Design review of the part built by this model. Coordinates are the model's own, in mm. A direction names the side the tool comes from. Round coordinates to 2 decimals unless told otherwise and drop trailing zeros. Order: outer loops, then holes, each group sorted by start corner. A loop starts at its lowest first (then second) coordinate and runs counter-clockwise, first axis right, second up. Notation, with made-up numbers: M -29.5,-7 L 20.5,-7 A33 cw 20.5,25 Z; hole C -33,85 d4. An arc over 180 degrees is marked long. Use a Markdown table: item, result. Add a question column.
(1) Take a section at C-C (z = 0). Write out the cut boundary in (x, y) (3 decimals), then the cut area to 3 significant figures.
(2) Take a section at D-D (x = -12). Write out the cut boundary in (y, z) (1 decimal), then the cut area to 3 significant figures.
(3) To check wall thickness, follow probe 1 along X at (y, z) = (3.5, 11.5) (1 decimal); probe 2 along X at (y, z) = (7.5, -12) (1 decimal); probe 3 along X at (y, z) = (8.25, 10.5) (1 decimal). State the ranges of each line that lie inside material, in increasing order. Write a range as from..to.
(4) Machinability: for faces 4 (the face through (-7.937, 5, -19)), 5 (the face through (9.68, 4.7, 8.34)), 6 (the face through (-3.175, 5, -13)), which of the approach directions +Z, -Z, +X, -X, +Y, -Y give a long, thin tool a straight path to every point of the face, cutting with its end or side? Answer none if there is none.
(5) For pin 1 (4 mm diameter, centred on y = 3.5, z = -0.5, fed in from +X); pin 2 (3 mm diameter, centred on y = 4.76, z = -15.88, fed in from +X); pin 3 (3 mm diameter, centred on y = 5, z = -12.5, fed in from +X); pin 4 (1.3 mm diameter, centred on x = 13.5, y = 4.5, fed in from -Z) (3 decimals), all flat-tipped, find the tip position at first contact; note any pin that passes through.
(6) The part is to be moulded in two halves that separate along Z. For faces 1 (the face through (13.46, 2.407, 15.352)), 2 (the face through (11.112, 5.9, 18.2)), 3 (the face through (-6, 5, -22.225)), say which applies: released by +Z, released by -Z, zero draft, split by the parting line, or undercut.
(7) Take a section at B-B (x = 0). Write out the cut boundary in (y, z) (3 decimals).
```python
from build123d import *

# Parameters (mm, degrees)
BOSS_EXTRUDE1_DEPTH                   = 9.525
SKETCH2_W                             = 19.05
SKETCH2_H                             = 15.24
SKETCH2_W_2                           = 22.225
CUT_EXTRUDE1_DEPTH                    = 10.525
F_3_16_0_1875_CLEARANCE_DOWEL_HOLE1_D = 4.826
F_10_24_TAPPED_HOLE1_D                = 3.7973
F_10_24_TAPPED_HOLE1_DEPTH            = 9.525
FILLET1_R                             = 4.7625
FILLET2_R                             = 12.7


with BuildPart() as part:
    # Sketch1 → Boss-Extrude1 (new body)
    with BuildSketch(Plane(origin=(0, 0, 0), x_dir=(1, 0, 0), z_dir=(0, 1, 0))):
        Polygon((-3.175, 22.225), (-3.175, 6.985), (3.175, 6.985), (3.175, 22.225), (26.9875, 22.225), (26.9875, -22.225), (22.225, -22.225), (22.225, -6.985), (15.875, -6.985), (15.875, -22.225), (-15.875, -22.225), (-15.875, -6.985), (-22.225, -6.985), (-22.225, -22.225), (-26.9875, -22.225), (-26.9875, 22.225), align=None)
    extrude(amount=BOSS_EXTRUDE1_DEPTH)

    # Sketch2 → Cut-Extrude1 (cut, through all)
    with BuildSketch(Plane(origin=(0, 9.525, 0), x_dir=(1, 0, 0), z_dir=(0, 1, 0))):
        with Locations((-17.4625, 14.605)):
            Rectangle(SKETCH2_W, SKETCH2_H)
        with Locations((17.4625, 14.605)):
            Rectangle(SKETCH2_W, SKETCH2_H)
        with Locations((0, -14.605)):
            Rectangle(SKETCH2_W_2, SKETCH2_H)
    extrude(amount=-CUT_EXTRUDE1_DEPTH, mode=Mode.SUBTRACT)

    # 3/16 (0.1875) Clearance Dowel Hole1 (through all)
    with Locations(Plane(origin=(26.9875, 0, 0), x_dir=(0, 0, -1), z_dir=(1, 0, 0))):
        with Locations((-15.875, 4.7625), (15.875, 4.7625)):
            Hole(F_3_16_0_1875_CLEARANCE_DOWEL_HOLE1_D / 2)

    # #10-24 Tapped Hole1
    with Locations(Plane(origin=(0, 9.525, 0), x_dir=(1, 0, 0), z_dir=(0, 1, 0))):
        with Locations((0, 0)):
            Hole(F_10_24_TAPPED_HOLE1_D / 2, depth=F_10_24_TAPPED_HOLE1_DEPTH)

    # Fillet1
    fillet1_edges = [part.edges().sort_by_distance(p)[0] for p in [
        (-7.9375, 4.7625, -6.985),
        (7.9375, 4.7625, -6.985),
        (-11.1125, 4.7625, 6.985),
        (11.1125, 4.7625, 6.985),
    ]]
    fillet(fillet1_edges, radius=FILLET1_R)

    # Fillet2
    fillet2_edges = [part.edges().sort_by_distance(p)[0] for p in [
        (-26.9875, 4.7625, -6.985),
        (26.9875, 4.7625, -6.985),
    ]]
    fillet(fillet2_edges, radius=FILLET2_R)


solid = part.part
```
Verdict:
| question | item | result |
|---|---|---|
| 1 | outline | M -25.629,0 L -1.899,0 L -1.899,9.525 L -25.629,9.525 Z; M 1.899,0 L 25.629,0 L 25.629,9.525 L 1.899,9.525 Z |
| 1 | area | 452 mm^2 |
| 2 | outline | M 0,-7 L 9.5,-7 L 9.5,22.2 L 0,22.2 Z; hole C 4.8,15.9 d4.8 |
| 2 | area | 260 mm^2 |
| 3 | probe 1 | x = -27..-22.2, -15.9..-11.1, 11.1..15.9, 22.2..27 |
| 3 | probe 2 | x = -7.9..-3.2, 3.2..7.9 |
| 3 | probe 3 | x = -27..-22.2, -15.9..-10.9, 10.9..15.9, 22.2..27 |
| 4 | face 4 | -Z, -X, +Y, -Y |
| 4 | face 5 | +Z, +Y, -Y |
| 4 | face 6 | -Z, +Y, -Y |
| 5 | pin 1 | stops at x = 26.27 |
| 5 | pin 2 | passes through |
| 5 | pin 3 | stops at x = 8 |
| 5 | pin 4 | stops at z = -6.985 |
| 6 | face 1 | undercut |
| 6 | face 2 | zero draft |
| 6 | face 3 | released by -Z |
| 7 | outline | M 0,-6.985 L 9.525,-6.985 L 9.525,-1.899 L 0,-1.899 Z; M 0,1.899 L 9.525,1.899 L 9.525,6.985 L 0,6.985 Z |
